Geometry: final body of the model. Coordinates: model frame, mm. Face numbers are marked on the shaded views. A direction names the side the tool comes from. Coordinates: 2 decimals unless noted, no trailing zeros. Loops run counter-clockwise (first coordinate to the right, second up) from the corner with the lowest first, then second, coordinate; pieces in that order, holes last. Notation, with made-up numbers: (86.25, 7) - (102.25, 7) arc R15 ccw to (102.25, 14) - close; hole circle Ø4 at (85, -12.5). An arc over 180 degrees is marked (long way). Put each result on its own line as item: value. Start each with the question number.
1) Contact query for flat-ended pins moving along their axis: pin 1 Ø3 at (y, z) = (89.5, 25.5) entering from -X; pin 2 Ø6 at (x, y) = (94, 65) entering from +Z; pin 3 Ø0.8 at (x, z) = (18, 24.5) entering from +Y; pin 4 Ø4 at (y, z) = (73, 28.5) entering from +X. Output: stop coordinate, or through.
2) Reachability of the marked faces 5, 6, 7 and 8 from +Z, -Z, +X, -X, +Y, -Y: full face, straight path, thin tool, end or side. Return the list, or none.
3) Draft query along X for the marked faces 1, 2, 3 and 4. Return one class per face: +X half, -X half, draft (parallel to the pull), parting line (faces both ways), or undercut.
4) Section D-D on y = 105.5. Output: boundary loops of the cut face in (x, z).
5) Section B-B on z = 29. Output: boundary loops of the cut face in (x, y), and give its area (3 significant figures).
6) Section C-C on x = 36. Output: boundary loops of the cut face in (y, z), and give its area (3 significant figures).
7) Section A-A on y = 26.5. Output: boundary loops of the cut face in (x, z), and give its area (3 significant figures).
8) Material intervals for line 1 along X through (y, z) = (16, 29.5); line 2 along Y through (x, z) = (-87, 13.5); line 3 along Z through (x, y) = (95.5, 99), sorted ascending. Write a range as from..to.
```python
from build123d import *

# Parameters (mm, degrees)
PAD004_DEPTH    = 25
SKETCH007_W     = 20
SKETCH007_H     = 22
PAD005_DEPTH    = 16
FILLET003_R     = 2
SKETCH010_W     = 172
SKETCH010_H     = 20
POCKET003_DEPTH = 16
FILLET007_R     = 15
FILLET008_R     = 5
FILLET009_R     = 1


with BuildPart() as part:
    # Sketch006 → Pad004 (new body)
    with BuildSketch(Plane.XY):
        Polygon((-108, 42), (-88, 42), (-88, 22), (88, 22), (88, 137), (108, 137), (108, 0), (-108, 0), align=None)
    extrude(amount=PAD004_DEPTH)

    # Sketch007 (on DatumPlane) → Pad005 (join)
    with BuildSketch(Plane.XY.offset(25)):
        with Locations((-98, 11)):
            Rectangle(SKETCH007_W, SKETCH007_H)
        with Locations((98, 11)):
            Rectangle(SKETCH007_W, SKETCH007_H)
    extrude(amount=PAD005_DEPTH)

    # Fillet003
    fillet003_edges = [part.edges().sort_by_distance(p)[0] for p in [
        (-98, 42, 0),
        (-88, 32, 0),
        (0, 22, 0),
        (88, 79.5, 0),
        (98, 137, 0),
        (108, 68.5, 0),
        (0, 0, 0),
        (-108, 21, 0),
    ]]
    fillet(fillet003_edges, radius=FILLET003_R)

    # Sketch010 (on DatumPlane) → Pocket003 (cut)
    with BuildSketch(Plane.XY.offset(25)):
        with Locations((0, 12)):
            Rectangle(SKETCH010_W, SKETCH010_H)
    extrude(amount=-POCKET003_DEPTH, mode=Mode.SUBTRACT)

    # Fillet007
    fillet007_edges = [part.edges().sort_by_distance(p)[0] for p in [
        (0, 2, 9),
    ]]
    fillet(fillet007_edges, radius=FILLET007_R)

    # Fillet008
    fillet008_edges = [part.edges().sort_by_distance(p)[0] for p in [
        (-98, 22, 41),
        (98, 22, 41),
    ]]
    fillet(fillet008_edges, radius=FILLET008_R)

    # Fillet009
    fillet009_edges = [part.edges().sort_by_distance(p)[0] for p in [
        (108, 0, 33),
        (108, 0, 13.5),
        (-108, 0, 33),
        (-108, 0, 13.5),
    ]]
    fillet(fillet009_edges, radius=FILLET009_R)


solid = part.part
```
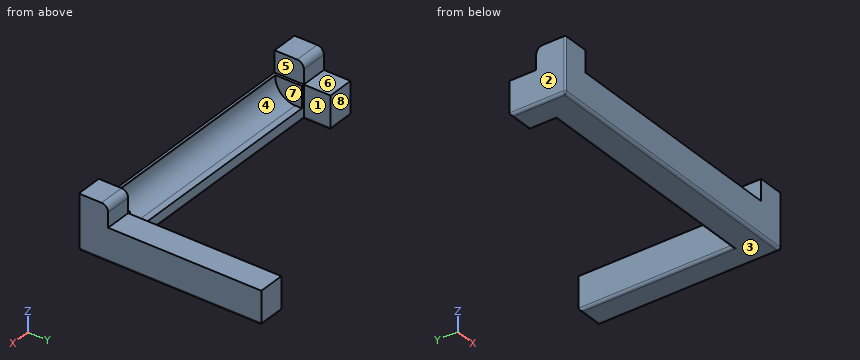
Answer block:
1. pin 1: stops at x = 88
1. pin 2: stops at z = 25
1. pin 3: stops at y = 2
1. pin 4: passes through
2. face 5: +Z, +Y, -Y
2. face 6: +Z, +X, -X, +Y
2. face 7: +Z, +Y
2. face 8: +Z, -Z, -X, +Y
3. face 1: undercut
3. face 2: -X half
3. face 3: draft
3. face 4: undercut
4. outline: (88, 2) arc R2 ccw to (90, 0) - (106, 0) arc R2 ccw to (108, 2) - (108, 25) - (88, 25) - close
5. outline: (-108, 1) arc R1 ccw to (-107, 0) - (-88, 0) - (-88, 22) - (-108, 22) - close; (88, 0) - (107, 0) arc R1 ccw to (108, 1) - (108, 22) - (88, 22) - close
5. area: 880 mm²
6. outline: (0, 2) arc R2 ccw to (2, 0) - (20, 0) arc R2 ccw to (22, 2) - (22, 9) - (17, 9) arc R15 cw to (2, 24) - (2, 25) - (0, 25) - close
6. area: 277 mm²
7. outline: (-108, 2) arc R2 ccw to (-106, 0) - (-90, 0) arc R2 ccw to (-88, 2) - (-88, 25) - (-108, 25) - close; (88, 2) arc R2 ccw to (90, 0) - (106, 0) arc R2 ccw to (108, 2) - (108, 25) - (88, 25) - close
7. area: 997 mm²
8. line 1: x = -108..-88, 88..108
8. line 2: y = 0..22
8. line 3: z = 0..25
